Could you check a few things on this drawing? It's one solid part, dimensions in mm from its lowest x, y, z. A direction names the side the tool comes from. Round coordinates to 2 decimals unless told otherwise and drop trailing zeros. Loops run counter-clockwise (first coordinate to the right, second up) from the corner with the lowest first, then second, coordinate; pieces in that order, holes last. Notation, with made-up numbers: M -24,-21 L -14,-21 A19 ccw -14,-4 Z; hole C 40.5,2.25 d1. An arc over 180 degrees is marked long. Write item = value, one per line. Start each with the question number.
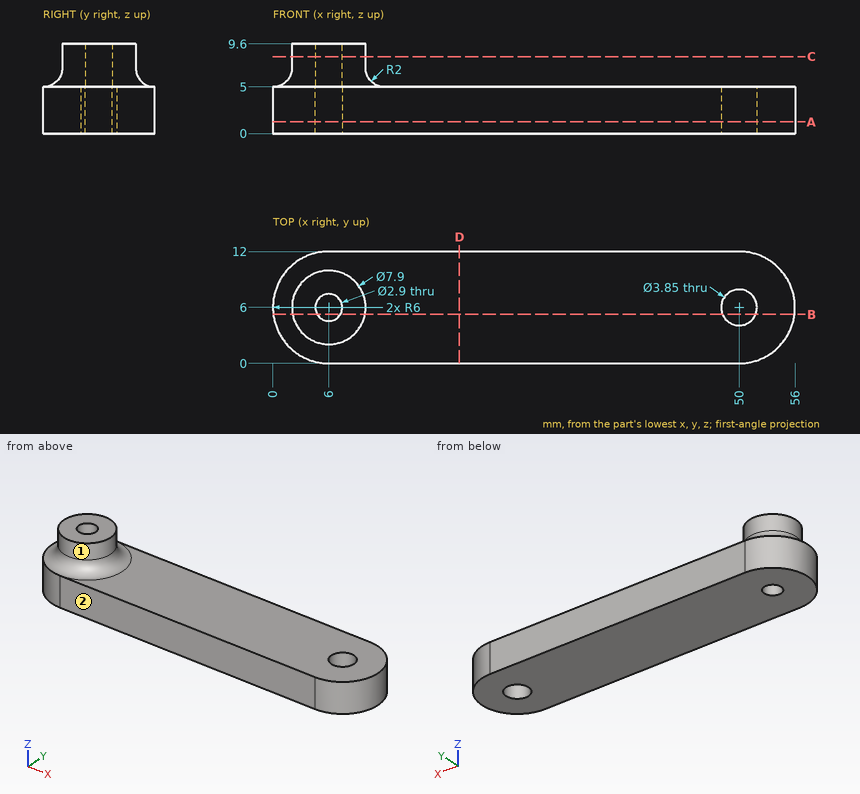
Item 1: I want a section at D-D, the plane x = 20. List the corners of the cut face in (y, z) for me.
Item 2: Will these pins go through, and if not, where does the flat tip stop? pin 1 Ø5 at (y, z) = (1.5, 2) entering from -X; pin 2 Ø2 at (x, y) = (24, 7) entering from +Z.
Item 3: I want a section at C-C, the plane z = 8.25. List the corners of the cut face in (x, y) for me.
Item 4: I want a section at B-B, the plane y = 5.25. State how many separate pieces and enclosed holes the cut face has, then the cut area to 3 significant figures.
Item 5: Please list where these lines run through material, in increasing order: line 1 (Y direction, x = 6, z = 1.55); line 2 (Y direction, x = 6, z = 8); line 3 (X direction, y = 5.75, z = 4.75). Write a range as [from, to].
Item 6: For the marked faces 1 and 2, which set-ups out of +Z, -Z, +X, -X, +Y, -Y let a thin tool reach every point of the face, with its end or its side?
Item 7: I want a section at A-A, the plane z = 1.25. List the corners of the cut face in (x, y) for me (3 decimals), then the cut area to 3 significant figures.
Worked out:
q1.outline = M 0,0 L 12,0 L 12,5 L 0,5 Z
q2.pin_1 = 0.34
q2.pin_2 = 5
q3.outline = C 6,6 d7.9; hole C 6,6 d2.9
q4.separate_pieces = 3
q4.enclosed_holes = 0
q4.area = 275 mm2
q5.line_1 = [0, 4.55], [7.45, 12]
q5.line_2 = [2.05, 4.55], [7.45, 9.95]
q5.line_3 = [0.01, 4.57], [7.43, 48.09], [51.91, 55.99]
q6.face_1 = +Z
q6.face_2 = +Z, -Z, +X, -X, -Y
q7.outline = M 6,0 L 50,0 A6 ccw 50,12 L 6,12 A6 ccw Z; hole C 6,6 d2.9; hole C 50,6 d3.85
q7.area = 623 mm2
